from build123d import *

# Parameters (mm, degrees)
SKETCH1_W           = 50.8
SKETCH1_H           = 76.2
BOSS_EXTRUDE1_DEPTH = 2.9972
SKETCH2_W           = 2.9972
SKETCH2_H           = 12.7
BOSS_EXTRUDE2_DEPTH = 2.9972
SKETCH3_W           = 38.1
SKETCH3_H           = 63.5
CUT_EXTRUDE1_DEPTH  = 48.612962265
EXTRUDE_THIN1_DEPTH = 2.9972
FILLET1_R           = 1.5875


with BuildPart() as part:
    # Sketch1 → Boss-Extrude1 (new body)
    with BuildSketch(Plane(origin=(0, 0, 0), x_dir=(1, 0, 0), z_dir=(0, 1, 0))):
        Rectangle(SKETCH1_W, SKETCH1_H)
    extrude(amount=BOSS_EXTRUDE1_DEPTH)

    # Sketch2 → Boss-Extrude2 (add)
    with BuildSketch(Plane(origin=(0, 2.9972, 0), x_dir=(1, 0, 0), z_dir=(0, 1, 0))):
        with Locations((26.8986, 0)):
            Rectangle(SKETCH2_W, SKETCH2_H)
        with Locations((26.8986, 31.75)):
            Rectangle(SKETCH2_W, SKETCH2_H)
        with Locations((26.8986, -31.75)):
            Rectangle(SKETCH2_W, SKETCH2_H)
        with Locations((-26.8986, 0)):
            Rectangle(SKETCH2_W, SKETCH2_H)
        with Locations((-26.8986, -31.75)):
            Rectangle(SKETCH2_W, SKETCH2_H)
        with Locations((-26.8986, 31.75)):
            Rectangle(SKETCH2_W, SKETCH2_H)
    extrude(amount=-BOSS_EXTRUDE2_DEPTH)

    # Sketch3 → Cut-Extrude1 (cut, through all)
    with BuildSketch(Plane(origin=(0, 2.9972, 0), x_dir=(1, 0, 0), z_dir=(0, 1, 0))):
        Rectangle(SKETCH3_W, SKETCH3_H)
    extrude(amount=-CUT_EXTRUDE1_DEPTH, mode=Mode.SUBTRACT)

    # Sketch4 → Extrude-Thin1 (add)
    with BuildSketch(Plane(origin=(0, 2.9972, 0), x_dir=(1, 0, 0), z_dir=(0, 1, 0))):
        Polygon((-21.082585469, 29.310897437), (14.090491456, 0), (-21.082585469, -29.310897437), (-17.017414531, -34.189102563), (24.009508544, 0), (-17.017414531, 34.189102563), align=None)
        Polygon((21.082585469, -29.310897437), (-14.090491456, 0), (21.082585469, 29.310897437), (17.017414531, 34.189102563), (-24.009508544, 0), (17.017414531, -34.189102563), align=None)
    extrude(amount=-EXTRUDE_THIN1_DEPTH)

    # Fillet1
    fillet1_edges = [part.edges().sort_by_distance(p)[0] for p in [
        (14.090491456, 1.4986, 31.75),
        (-14.090491456, 1.4986, 31.75),
        (19.05, 1.4986, -27.617076213),
        (19.05, 1.4986, 27.617076213),
        (19.05, 1.4986, 4.132923787),
        (19.05, 1.4986, -4.132923787),
        (14.090491456, 1.4986, -31.75),
        (-14.090491456, 1.4986, -31.75),
        (-19.05, 1.4986, -4.132923787),
        (-19.05, 1.4986, 4.132923787),
        (-19.05, 1.4986, -27.617076213),
        (-19.05, 1.4986, 27.617076213),
        (-4.959508544, 1.4986, 15.875),
        (-4.959508544, 1.4986, -15.875),
        (0, 1.4986, -20.007923787),
        (4.959508544, 1.4986, -15.875),
        (4.959508544, 1.4986, 15.875),
        (0, 1.4986, 20.007923787),
        (14.090491456, 1.4986, 0),
        (0, 1.4986, -11.742076213),
        (0, 1.4986, 11.742076213),
        (-14.090491456, 1.4986, 0),
    ]]
    fillet(fillet1_edges, radius=FILLET1_R)


solid = part.part
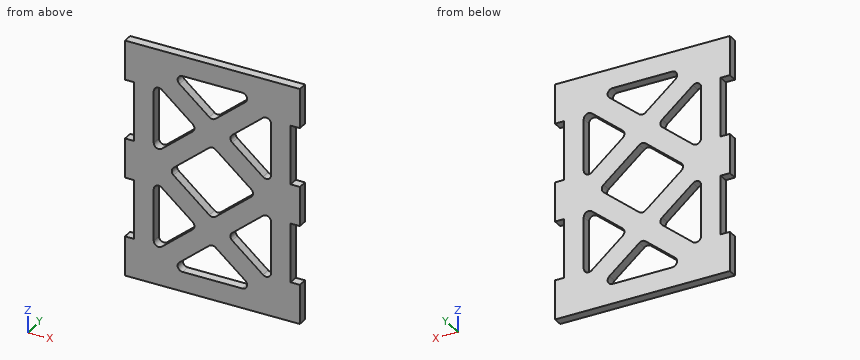
Source: CAD feature listing. Evaluate the final solid. Frame: model axes, mm. Give positions to 0.01 mm unless a question says otherwise; leave off trailing zeros. Write each loop counter-clockwise with the first axis right and the second up, starting at its lowest first coordinate (ties: lowest second). Pieces come first, ordered by that corner, then holes. Notation, with made-up numbers: (74.5, 85) -> (97.5, 85) arc R25 cw to (97.5, 107) -> close; hole circle Ø10 at (-22.75, -23). An arc over 180 degrees is marked (long way). Write item = value, one per line.
Q1. Line query: line 1 (Z direction, x = -25.5, y = 1.7); line 2 (X direction, y = 1.85, z = -16); line 3 (Z direction, x = 11, y = 0.4). Output: solid intervals per line, ascending. Write a range as from..to.
Here are the results:
line_1 = -38.1..-25.4, -6.35..6.35, 25.4..38.1
line_2 = -25.4..-19.05, -5.86..5.86, 19.05..25.4
line_3 = -38.1..-31.08, -29.24..-20.91, -10.84..-2.58, 2.58..10.84, 20.91..29.24, 31.08..38.1
Q2. Cut plane B-B on z = -30.5. Return loops of the section in (x, y), then the cut area to 3 significant figures.
Here are the results:
outline = (-28.4, 0) -> (-11.26, 0) -> (-11.26, 3) -> (-28.4, 3) -> close; (11.26, 0) -> (28.4, 0) -> (28.4, 3) -> (11.26, 3) -> close
area = 103 mm²
Q3. Cut plane C-C on x = -18. Return loops of the section in (y, z), then the cut area to 3 significant figures.
Here are the results:
outline = (0, -38.1) -> (3, -38.1) -> (3, -25.72) -> (0, -25.72) -> close; (0, -6.03) -> (3, -6.03) -> (3, 6.03) -> (0, 6.03) -> close; (0, 25.72) -> (3, 25.72) -> (3, 38.1) -> (0, 38.1) -> close
area = 110 mm²
Q4. Cut plane D-D on x = -7.5. Return loops of the section in (y, z), then the cut area to 3 significant figures.
Here are the results:
outline = (0, -38.1) -> (3, -38.1) -> (3, -31.75) -> (0, -31.75) -> close; (0, -26.26) -> (3, -26.26) -> (3, -17.99) -> (0, -17.99) -> close; (0, -13.76) -> (3, -13.76) -> (3, -5.49) -> (0, -5.49) -> close; (0, 5.49) -> (3, 5.49) -> (3, 13.76) -> (0, 13.76) -> close; (0, 17.99) -> (3, 17.99) -> (3, 26.26) -> (0, 26.26) -> close; (0, 31.75) -> (3, 31.75) -> (3, 38.1) -> (0, 38.1) -> close
area = 137 mm²
Q5. Cut plane A-A on x = 4. Return loops of the section in (y, z), then the cut area to 3 significant figures.
Here are the results:
outline = (0, -38.1) -> (3, -38.1) -> (3, -31.75) -> (0, -31.75) -> close; (0, -23.34) -> (3, -23.34) -> (3, -8.41) -> (0, -8.41) -> close; (0, 8.41) -> (3, 8.41) -> (3, 23.34) -> (0, 23.34) -> close; (0, 31.75) -> (3, 31.75) -> (3, 38.1) -> (0, 38.1) -> close
area = 128 mm²
Q6. First-contact query: pin 1 (0.9 mm diameter, centred on y = 1.5, z = 20, fed in from +X); pin 2 (1.5 mm diameter, centred on y = 1, z = -18.5, fed in from -X). Flat tips, straight axial feed; report the tip coordinate or a pass-through.
Here are the results:
pin_1 = 25.4
pin_2 = -25.4
